Build history of the part. All positions in model axes, mm. Face numbers are marked on the shaded views. Round coordinates to 2 decimals unless told otherwise and drop trailing zeros. Loops run counter-clockwise (first coordinate to the right, second up) from the corner with the lowest first, then second, coordinate; pieces in that order, holes last. Notation, with made-up numbers: (-33, -5.75) -> (12, -5.75) arc R27 cw to (12, 11.25) -> close; hole circle Ø5 at (69, 89). An arc over 180 degrees is marked (long way). Put each result on its own line as item: value. Start each with the question number.
Item 1: Cut at D-D, the plane y = -93.5. List the corners of the cut face in (x, z), plus the area to 3 significant figures.
Item 2: Drill centre lines: probe 1 along Y at (x, z) = (0, 119) (3 decimals); probe 2 along Y at (x, z) = (0, -3) (3 decimals); probe 3 along X at (y, z) = (7, 62). Where is each one in solid material? Low to high. Write a range as [from, to].
Item 3: Pull direction X, two halves, no side cores. Call the marked faces 1, 2, 3 and 4: +X half, -X half, draft (parallel to the pull), parting line (faces both ways), or undercut.
Item 4: Cut at C-C, the plane z = 61. List the corners of the cut face in (x, y) (3 decimals), plus the area to 3 significant figures.
Item 5: Cut at A-A, the plane y = 0. List the corners of the cut face in (x, z) (3 decimals), plus the area to 3 significant figures.
Item 6: Flat gauge pins, fed straight in: pin 1 Ø3 at (x, y) = (-59.5, 78) entering from +Z; pin 2 Ø8 at (x, z) = (121.5, 56.5) entering from +Y; pin 3 Ø1.5 at (x, z) = (-136.5, 65.5) entering from +Y. Where does each tip first touch, or does it go through?
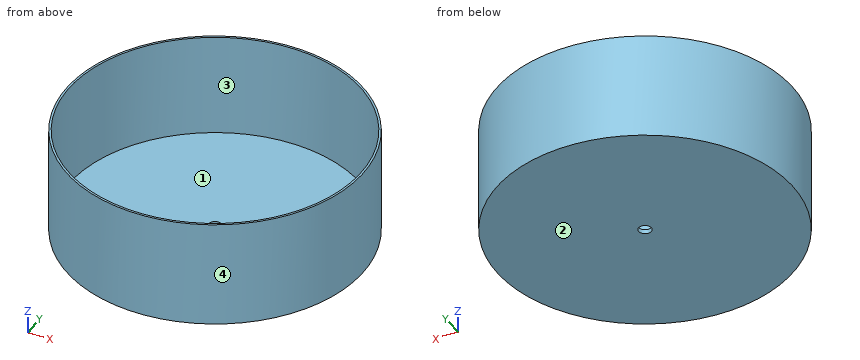
```python
from build123d import *

# Parameters (mm, degrees)
F0_R     = 219.075
F0_R_2   = 215.9
F1_DEPTH = 152.4
F2_R     = 219.075
F3_DEPTH = 6.35
F4_R     = 9.525
F5_DEPTH = 25.4


with BuildPart() as f1:
    # F0 (on Top) → F1 (new body)
    with BuildSketch(Plane.XY):
        Circle(F0_R)
        Circle(F0_R_2, mode=Mode.SUBTRACT)
    extrude(amount=F1_DEPTH)

    # F2 (on Top) → F3 (join)
    with BuildSketch(Plane.XY):
        Circle(F2_R)
    extrude(amount=-F3_DEPTH)

    # F4 (on face) → F5 (cut)
    with BuildSketch(Plane(origin=(0, 0, -6.35), x_dir=(1, 0, 0), z_dir=(0, 0, -1))):
        Circle(F4_R)
    extrude(amount=-F5_DEPTH, mode=Mode.SUBTRACT)


solid = f1.part
```
Reply:
1. outline: (-198.12, -6.35) -> (198.12, -6.35) -> (198.12, 152.4) -> (194.6, 152.4) -> (194.6, 0) -> (-194.6, 0) -> (-194.6, 152.4) -> (-198.12, 152.4) -> close
1. area: 3,590 mm^2
2. probe 1: y = [-219.075, -215.9], [215.9, 219.075]
2. probe 2: y = [-219.075, -9.525], [9.525, 219.075]
2. probe 3: x = [-218.96, -215.79], [215.79, 218.96]
3. face 1: undercut
3. face 2: draft
3. face 3: undercut
3. face 4: parting line
4. outline: circle Ø438.15 at (0, 0); hole circle Ø431.8 at (0, 0)
4. area: 4,340 mm^2
5. outline: (-219.075, -6.35) -> (-9.525, -6.35) -> (-9.525, 0) -> (-215.9, 0) -> (-215.9, 152.4) -> (-219.075, 152.4) -> close; (9.525, -6.35) -> (219.075, -6.35) -> (219.075, 152.4) -> (215.9, 152.4) -> (215.9, 0) -> (9.525, 0) -> close
5. area: 3,630 mm^2
6. pin 1: stops at z = 0
6. pin 2: stops at y = 184.9
6. pin 3: stops at y = 171.95
